Here's how the part is built. I have some questions about the finished solid (model axes, mm). A direction names the side the tool comes from. Give positions to 0.01 mm unless a question says otherwise; leave off trailing zeros. Order: outer loops, then holes, each group sorted by start corner. A loop starts at its lowest first (then second) coordinate and runs counter-clockwise, first axis right, second up. Notation, with made-up numbers: M -3.5,-37 L 43.5,-37 A12 ccw 43.5,-33 Z; hole C 16.25,-8.5 d11. An arc over 180 degrees is marked long. One line per item, written item: value. Start each with the question number.
from build123d import *

# Parameters (mm, degrees)
BOSS_EXTRUDE1_DEPTH = 38.1
SKETCH2_W           = 81.28
SKETCH2_H           = 34.925
SKETCH2_W_2         = 74.676
SKETCH2_H_2         = 28.321
CUT_EXTRUDE1_DEPTH  = 3.302


with BuildPart() as part:
    # Sketch1 → Boss-Extrude1 (new body)
    with BuildSketch(Plane.XY):
        Polygon((-50.8, 0), (-50.8, -6.35), (-41.275, -6.35), (-41.275, -38.1), (41.275, -38.1), (41.275, -6.35), (50.8, -6.35), (50.8, 0), align=None)
    extrude(amount=BOSS_EXTRUDE1_DEPTH)

    # Sketch2 → Cut-Extrude1 (cut)
    with BuildSketch(Plane(origin=(0, 0, 0), x_dir=(1, 0, 0), z_dir=(0, 1, 0))):
        with Locations((0, -19.05)):
            Rectangle(SKETCH2_W, SKETCH2_H)
        with Locations((0, -19.05)):
            Rectangle(SKETCH2_W_2, SKETCH2_H_2, mode=Mode.SUBTRACT)
    extrude(amount=-CUT_EXTRUDE1_DEPTH, mode=Mode.SUBTRACT)


solid = part.part
Item 1: Please list where these lines run through material, in increasing order: probe 1 along Z at (x, y) = (-30.5, -2.5); probe 2 along X at (y, z) = (-3, 32.5); probe 3 along X at (y, z) = (-10, 20) (3 decimals). Write a range as [from, to].
Item 2: For faces 5 (the face through (-41.275, -22, 19)), 6 (the face through (50.8, -3, 19)), 7 (the face through (-1, -2, 36.512)), which set-ups out of +Z, -Z, +X, -X, +Y, -Y let a thin tool reach every point of the face, with its end or its side?
Item 3: I want a section at C-C on y = -16. Write out the boundary of the cut face in (x, z) (3 decimals).
Item 4: I want a section at A-A on x = 19. Write out the boundary of the cut face in (y, z).
Item 5: Will these pins go through, and if not, where does the flat tip stop? P1, Ø9.5, axis at y = -18.5, z = 21, coming from the -X side (3 decimals); P2, Ø3, axis at x = 48, z = 23.5, coming from the -Y side; P3, Ø1, axis at y = -29, z = 12.5, coming from the +X side (3 decimals).
Item 6: I want a section at B-B on z = 9.5. Write out the boundary of the cut face in (x, y) (3 decimals), plus the area to 3 significant figures.
Item 7: We'd pull the mould along X, two halves only. Please class faces 1 (the face through (1, 0, 19)), 2 (the face through (-1, -2, 4.89)), 3 (the face through (41.275, -22, 19)), 4 (the face through (40.64, -2, 19)): +X half, -X half, draft (parallel to the pull), parting line (faces both ways), or undercut.
Answer below:
1. probe 1: z = [0, 1.59], [4.89, 33.21], [36.51, 38.1]
1. probe 2: x = [-50.8, -40.64], [-37.34, 37.34], [40.64, 50.8]
1. probe 3: x = [-41.275, 41.275]
2. face 5: +Z, -Z, -X, -Y
2. face 6: +Z, -Z, +X, +Y, -Y
2. face 7: +Y
3. outline: M -41.275,0 L 41.275,0 L 41.275,38.1 L -41.275,38.1 Z
4. outline: M -38.1,0 L 0,0 L 0,1.59 L -3.3,1.59 L -3.3,4.89 L 0,4.89 L 0,33.21 L -3.3,33.21 L -3.3,36.51 L 0,36.51 L 0,38.1 L -38.1,38.1 Z
5. P1: stops at x = -41.275
5. P2: stops at y = -6.35
5. P3: stops at x = 41.275
6. outline: M -50.8,-6.35 L -41.275,-6.35 L -41.275,-38.1 L 41.275,-38.1 L 41.275,-6.35 L 50.8,-6.35 L 50.8,0 L 40.64,0 L 40.64,-3.302 L 37.338,-3.302 L 37.338,0 L -37.338,0 L -37.338,-3.302 L -40.64,-3.302 L -40.64,0 L -50.8,0 Z
6. area: 3,240 mm²
7. face 1: draft
7. face 2: undercut
7. face 3: +X half
7. face 4: undercut
